Input: dimensioned drawing with shaded views. Units: mm. Origin: part minimum x, y, z. A direction names the side the tool comes from. Coordinates: 2 decimals unless noted, no trailing zeros. Order: outer loops, then holes, each group sorted by start corner. A loop starts at its lowest first (then second) coordinate and runs counter-clockwise, first axis right, second up. Notation, with made-up numbers: (45, -25) -> (77, -25) arc R17 ccw to (77, -9) -> close; hole circle Ø7 at (58, 62.5). An arc over 180 degrees is marked (long way). Answer as CSV lines item,"result".
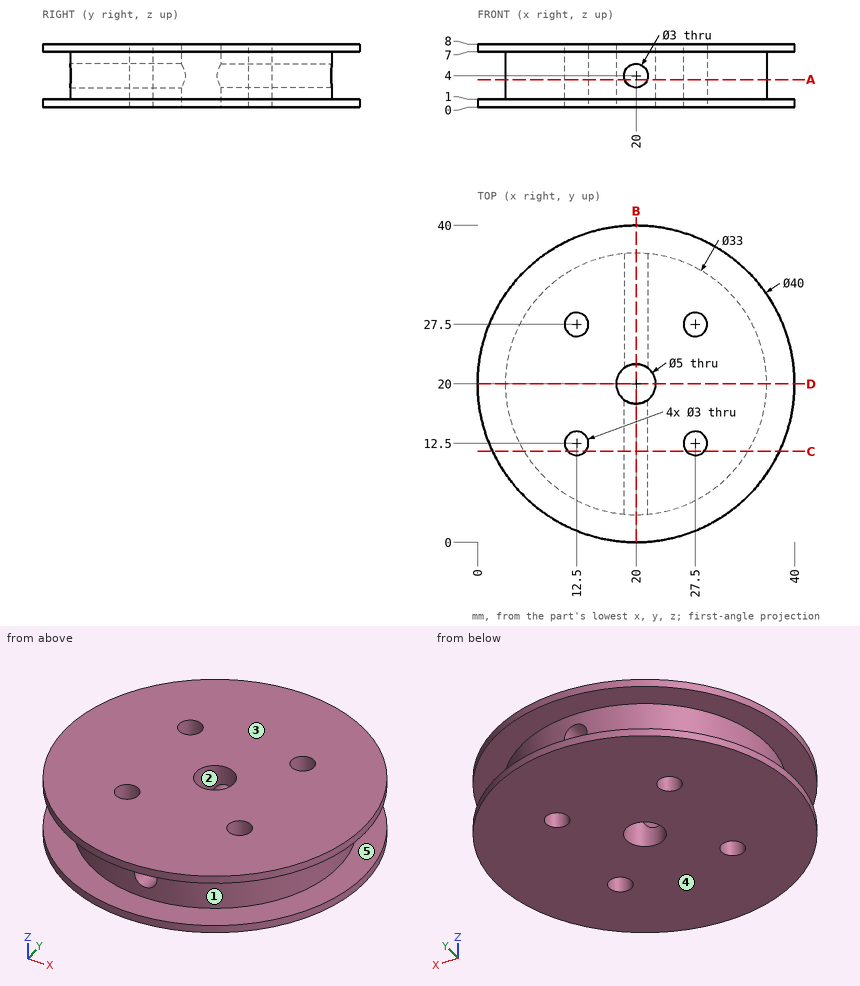
1. Reachability of the marked faces 1 and 2 from +Z, -Z, +X, -X, +Y, -Y: full face, straight path, thin tool, end or side. Return the list, or none.
Findings:
face 1,"none"
face 2,"+Z, -Z"
2. Cut plane C-C (y = 11.5). Return the cut outline in (x, z), plus the area to 3 significant figures.
Findings:
outline,"(1.9, 0) -> (11.38, 0) -> (11.38, 8) -> (1.9, 8) -> (1.9, 7) -> (5.86, 7) -> (5.86, 1) -> (1.9, 1) -> close; (13.62, 0) -> (26.38, 0) -> (26.38, 8) -> (13.62, 8) -> close; (28.62, 0) -> (38.1, 0) -> (38.1, 1) -> (34.14, 1) -> (34.14, 7) -> (38.1, 7) -> (38.1, 8) -> (28.62, 8) -> close; hole circle Ø3 at (20, 4)"
area,"199 mm2"
3. Cut plane D-D (y = 20). Return the cut outline in (x, z).
Findings:
outline,"(0, 0) -> (17.5, 0) -> (17.5, 8) -> (0, 8) -> (0, 7) -> (3.5, 7) -> (3.5, 1) -> (0, 1) -> close; (22.5, 0) -> (40, 0) -> (40, 1) -> (36.5, 1) -> (36.5, 7) -> (40, 7) -> (40, 8) -> (22.5, 8) -> close"
4. Cut plane B-B (x = 20). Return the cut outline in (y, z).
Findings:
outline,"(0, 0) -> (17.5, 0) -> (17.5, 2.5) -> (3.5, 2.5) -> (3.5, 1) -> (0, 1) -> close; (0, 7) -> (3.5, 7) -> (3.5, 5.5) -> (17.5, 5.5) -> (17.5, 8) -> (0, 8) -> close; (22.5, 0) -> (40, 0) -> (40, 1) -> (36.5, 1) -> (36.5, 2.5) -> (22.5, 2.5) -> close; (22.5, 5.5) -> (36.5, 5.5) -> (36.5, 7) -> (40, 7) -> (40, 8) -> (22.5, 8) -> close"
5. Mould query, pull axis Z, two halves, no side actions, for the marked faces 3, 4 and 5. Classes: released by +Z, released by -Z, zero draft, split by the parting line, or undercut.
Findings:
face 3,"released by +Z"
face 4,"released by -Z"
face 5,"undercut"
6. Cut plane A-A (z = 3.5). Return the cut outline in (x, y), plus the area to 3 significant figures.
Findings:
outline,"(18.59, 3.56) -> (18.59, 17.94) arc R2.5 cw to (18.59, 22.06) -> (18.59, 36.44) arc R16.5 ccw to start; (21.41, 3.56) arc R16.5 ccw to (21.41, 36.44) -> (21.41, 22.06) arc R2.5 cw to (21.41, 17.94) -> close; hole circle Ø3 at (12.5, 12.5); hole circle Ø3 at (12.5, 27.5); hole circle Ø3 at (27.5, 12.5); hole circle Ø3 at (27.5, 27.5)"
area,"728 mm2"
7. Contact query for flat-ended pins moving along their axis: pin 1 (3.5 mm diameter, centred on x = 20, z = 4, fed in from +Y); pin 2 (2 mm diameter, centred on y = 25, z = 1.5, fed in from -X); pin 3 (4 mm diameter, centred on x = 20.5, z = 7, fed in from +Y). Output: stop coordinate, or through.
Findings:
pin 1,"stops at y = 36.5"
pin 2,"stops at x = 0.43"
pin 3,"stops at y = 40"
8. Ray query, line 1 along Z through (x, y) = (36.5, 30.5); line 2 along Y through (x, z) = (12.5, 4.5); line 3 along Y through (x, z) = (28, 5.25). Return the intervals inside material, ascending.
Findings:
line 1,"z = 0 to 1, 7 to 8"
line 2,"y = 5.3 to 11, 14 to 26, 29 to 34.7"
line 3,"y = 5.57 to 11.09, 13.91 to 26.09, 28.91 to 34.43"
